from build123d import *

# Parameters (mm, degrees)
F0_W      = 231
F0_H      = 100
F1_DEPTH  = 36
F2_W      = 48
F2_H      = 23.5
F2_H_2    = 48.2
F3_DEPTH  = 35.8
F4_W      = 48
F4_H      = 1.2
F5_DEPTH  = 15
F6_W      = 48
F6_H      = 97.6
F6_W_2    = 81
F7_DEPTH  = 35.8
F8_R      = 2.4
F9_R      = 1.2
F10_W     = 145.4325905085
F10_H     = 144.5563584566
F11_DEPTH = 40
F12_R     = 2.4


with BuildPart() as f1:
    # F0 (on Top) → F1 (new body)
    with BuildSketch(Plane.XY):
        Rectangle(F0_W, F0_H)
    extrude(amount=F1_DEPTH)

    # F2 (on face) → F3 (cut)
    with BuildSketch(Plane.XY.offset(36)):
        with Locations((41.1, 37.05)):
            Rectangle(F2_W, F2_H)
        with Locations((90.3, 37.05)):
            Rectangle(F2_W, F2_H)
        with Locations((41.1, 12.35)):
            Rectangle(F2_W, F2_H)
        with Locations((90.3, 12.35)):
            Rectangle(F2_W, F2_H)
        with Locations((41.1, -24.7)):
            Rectangle(F2_W, F2_H_2)
        with Locations((90.3, -24.7)):
            Rectangle(F2_W, F2_H_2)
    extrude(amount=-F3_DEPTH, mode=Mode.SUBTRACT)

    # F4 (on face) → F5 (cut)
    with BuildSketch(Plane.XY.offset(36)):
        with Locations((41.1, 24.7)):
            Rectangle(F4_W, F4_H)
        with Locations((90.3, 24.7)):
            Rectangle(F4_W, F4_H)
    extrude(amount=-F5_DEPTH, mode=Mode.SUBTRACT)

    # F6 (on face) → F7 (cut)
    with BuildSketch(Plane.XY.offset(36)):
        with Locations((-90.3, 0)):
            Rectangle(F6_W, F6_H)
        with Locations((-24.6, 0)):
            Rectangle(F6_W_2, F6_H)
    extrude(amount=-F7_DEPTH, mode=Mode.SUBTRACT)

    # F8
    f8_edges = [f1.edges().sort_by_distance(p)[0] for p in [
        (-115.5, -50, 18),
        (-115.5, 50, 18),
        (115.5, 50, 18),
        (115.5, -50, 18),
    ]]
    fillet(f8_edges, radius=F8_R)

    # F9
    f9_edges = [f1.edges().sort_by_distance(p)[0] for p in [
        (-90.3, 48.8, 0.2),
        (-114.3, 0, 0.2),
        (-90.3, -48.8, 0.2),
        (-66.3, 0, 0.2),
        (-24.6, 48.8, 0.2),
        (-65.1, 0, 0.2),
        (-24.6, -48.8, 0.2),
        (15.9, 0, 0.2),
        (41.1, 25.3, 0.2),
        (65.1, 37.05, 0.2),
        (41.1, 48.8, 0.2),
        (17.1, 37.05, 0.2),
        (114.3, 37.05, 0.2),
        (90.3, 48.8, 0.2),
        (66.3, 37.05, 0.2),
        (90.3, 25.3, 0.2),
        (65.1, 12.35, 0.2),
        (41.1, 24.1, 0.2),
        (17.1, 12.35, 0.2),
        (41.1, 0.6, 0.2),
        (90.3, 0.6, 0.2),
        (114.3, 12.35, 0.2),
        (90.3, 24.1, 0.2),
        (66.3, 12.35, 0.2),
        (17.1, -24.7, 0.2),
        (41.1, -48.8, 0.2),
        (65.1, -24.7, 0.2),
        (41.1, -0.6, 0.2),
        (114.3, -24.7, 0.2),
        (90.3, -0.6, 0.2),
        (66.3, -24.7, 0.2),
        (90.3, -48.8, 0.2),
        (-114.3, 48.8, 18.1),
        (-65.1, 48.8, 18.1),
        (-66.3, 48.8, 18.1),
        (-66.3, -48.8, 18.1),
        (-114.3, -48.8, 18.1),
        (15.9, 48.8, 18.1),
        (15.9, -48.8, 18.1),
        (-65.1, -48.8, 18.1),
        (17.1, -48.8, 18.1),
        (17.1, 0.6, 18.1),
        (17.1, 25.3, 10.6),
        (17.1, 48.8, 18.1),
        (17.1, 24.1, 10.6),
        (17.1, -0.6, 18.1),
        (65.1, -0.6, 18.1),
        (65.1, -48.8, 18.1),
        (65.1, 24.1, 10.6),
        (65.1, 25.3, 10.6),
        (65.1, 48.8, 18.1),
        (66.3, 48.8, 18.1),
        (114.3, 48.8, 18.1),
        (114.3, 24.1, 10.6),
        (114.3, 25.3, 10.6),
        (66.3, 25.3, 10.6),
        (66.3, 24.1, 10.6),
        (66.3, 0.6, 18.1),
        (66.3, -0.6, 18.1),
        (114.3, -0.6, 18.1),
        (114.3, 0.6, 18.1),
        (114.3, -48.8, 18.1),
        (66.3, -48.8, 18.1),
    ]]
    fillet(f9_edges, radius=F9_R)

    # F10 (on face) → F11 (cut)
    with BuildSketch(Plane.XY.offset(36)):
        with Locations((-56.8162952542, -9.1554522514)):
            Rectangle(F10_W, F10_H)
    extrude(amount=-F11_DEPTH, mode=Mode.SUBTRACT)

    # F12
    f12_edges = [f1.edges().sort_by_distance(p)[0] for p in [
        (15.9, 50, 18),
        (15.9, -50, 18),
    ]]
    fillet(f12_edges, radius=F12_R)


solid = f1.part
The listing builds one solid part. Answer for the finished solid, in the listing's coordinates (mm). A direction names the side the tool comes from. Give positions to 0.01 mm unless a question says otherwise; leave off trailing zeros. Write each loop counter-clockwise with the first axis right and the second up, starting at its lowest first coordinate (ties: lowest second). Pieces come first, ordered by that corner, then holes. Notation, with made-up numbers: (37, 85) - (80, 85) arc R26 ccw to (80, 108) - close; hole circle Ø7 at (88, -38.75). An arc over 180 degrees is marked (long way). One line per question, with ' | ' between items. Start each with the question number.
1. Section B-B, the plane y = -8 is taken. Determine the outline of the cut face in (x, z), then the cut area to 3 significant figures.
2. Straight lines are drawn through the part: line 1 (X direction, y = 25.5, z = 23.5); line 2 (Y direction, x = 101, z = 19.5); line 3 (Y direction, x = 83, z = 24). For each, find the intervals that lie inside material, in ascending order.
3. Given P1, Ø1.8, axis at x = 38, y = 25, coming from the +Z side; P2, Ø1.5, axis at x = 26, y = 2.5, coming from the +Z side, each flat-ended and moving along its own axis, determine where each tip first touches the part or whether it passes through.
4. Section A-A, the plane x = 82 is taken. Determine the outline of the cut face in (y, z).
5. Determine the mould class of faces 3 (the face through (90, -24, 0.2)), 4 (the face through (65, 1, 0)), 5 (the face through (114.778, -49.316, 18.252)) for opening direction Y: +Y half, -Y half, draft (parallel to the pull), parting line (faces both ways), or undercut.
6. Section C-C, the plane z = 14.5 is taken. Count the separate pieces of the cut face and the enclosed holes in it, then the cut area to 3 significant figures.
7. For faces 1 (the face through (16.622, -49.316, 17.748)), 2 (the face through (41, 24.1, 11)), determine the directions among +Z, -Z, +X, -X, +Y, -Y from which every point of the face is accessible in a straight line to the end or side of a thin tool.
Result:
1) outline: (15.9, 0) - (115.5, 0) - (115.5, 36) - (114.3, 36) - (114.3, 1.4) arc R1.2 cw to (113.1, 0.2) - (67.5, 0.2) arc R1.2 cw to (66.3, 1.4) - (66.3, 36) - (65.1, 36) - (65.1, 1.4) arc R1.2 cw to (63.9, 0.2) - (18.3, 0.2) arc R1.2 cw to (17.1, 1.4) - (17.1, 36) - (15.9, 36) - close | area: 150 mm2
2) line 1: x = 15.9 to 17.1, 65.1 to 66.3, 114.3 to 115.5 | line 2: y = -50 to -48.8, -0.6 to 0.6, 24.1 to 25.3, 48.8 to 50 | line 3: y = -50 to -48.8, -0.6 to 0.6, 48.8 to 50
3) P1: stops at z = 21 | P2: stops at z = 0.2
4) outline: (-50, 0) - (50, 0) - (50, 36) - (48.8, 36) - (48.8, 1.4) arc R1.2 cw to (47.6, 0.2) - (26.5, 0.2) arc R1.2 cw to (25.3, 1.4) - (25.3, 21) - (24.1, 21) - (24.1, 1.4) arc R1.2 cw to (22.9, 0.2) - (1.8, 0.2) arc R1.2 cw to (0.6, 1.4) - (0.6, 36) - (-0.6, 36) - (-0.6, 1.4) arc R1.2 cw to (-1.8, 0.2) - (-47.6, 0.2) arc R1.2 cw to (-48.8, 1.4) - (-48.8, 36) - (-50, 36) - close
5) face 3: undercut | face 4: draft | face 5: -Y half
6) separate pieces: 1 | enclosed holes: 6 | area: 823 mm2
7) face 1: +Z, -Z, -X, -Y | face 2: +Z
